from build123d import *

# Parameters (mm, degrees)
F0_W     = 37.5
F0_H     = 30
F1_DEPTH = 60


with BuildPart() as f1:
    # F0 (on Front) → F1 (new body)
    with BuildSketch(Plane.XZ):
        with Locations((-18.75, -15)):
            Rectangle(F0_W, F0_H)
        with Locations((-18.75, 15)):
            Rectangle(F0_W, F0_H)
        with Locations((18.75, 15)):
            Rectangle(F0_W, F0_H)
        with Locations((18.75, -15)):
            Rectangle(F0_W, F0_H)
        Polygon((-75, 0), (-37.5, 0), (-37.5, 30), (0, 30), (0, 60), (-75, 60), align=None)
        Polygon((75, 0), (37.5, 0), (37.5, -30), (0, -30), (0, -60), (75, -60), align=None)
    extrude(amount=F1_DEPTH)


solid = f1.part
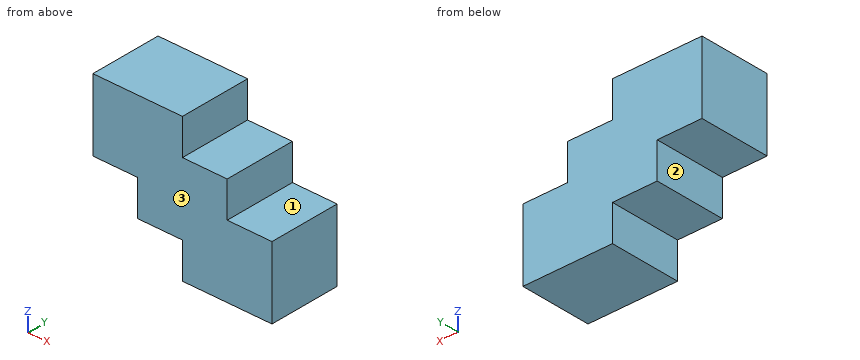
Input: part model. Units: mm. Frame: model coordinates. Face numbers are marked on the shaded views. A direction names the side the tool comes from. Coordinates: 2 decimals unless noted, no trailing zeros. Write each loop counter-clockwise with the first axis right and the second up, starting at its lowest first coordinate (ties: lowest second). Pieces come first, ordered by that corner, then holes. Notation, with made-up numbers: M -19.5,83 L 6.5,83 A24 cw 6.5,103 Z; hole C 28,11.5 d6. An arc over 180 degrees is marked long. Answer as a JSON object with one key per item and string values. Group by question number.
(1) Set-up query: the marked faces 1, 2 and 3. Return all of +Z, -Z, +X, -X, +Y, -Y with unobstructed straight access to the full face (end or side cutting, diameter ignored); none if empty.
(2) Section C-C on x = 24. Output: boundary loops of the cut face in (y, z).
(3) Contact query for flat-ended pins moving along their axis: P1, Ø24, axis at y = -23, z = 41.5, coming from the +X side; P2, Ø8, axis at y = -8, z = -33.5, coming from the -X side; P3, Ø3, axis at y = -20.5, z = 42.5, coming from the +X side. Output: stop coordinate, or through.
(4) Section A-A on y = -19. Output: boundary loops of the cut face in (x, z), plus the area to 4 significant figures.
(5) Ray query, line 1 along Z through (x, y) = (6, -41.5); line 2 along X through (y, z) = (-3, 7.5); line 3 along Z through (x, y) = (-58.5, -7). Return the intervals inside material, ascending. Write a range as [from, to].
(6) Section B-B on z = -49. Output: boundary loops of the cut face in (x, y).
Result set:
{
 "1": {"face 1": "+Z, +X, +Y, -Y", "face 2": "-Z, -X, +Y, -Y", "face 3": "+Z, -Z, +X, -X, -Y"},
 "2": {"outline": "M -60,-60 L 0,-60 L 0,30 L -60,30 Z"},
 "3": {"P1": "stops at x = 37.5", "P2": "stops at x = -37.5", "P3": "stops at x = 0"},
 "4": {"outline": "M -75,0 L -37.5,0 L -37.5,-30 L 0,-30 L 0,-60 L 75,-60 L 75,0 L 37.5,0 L 37.5,30 L 0,30 L 0,60 L -75,60 Z", "area": "11,250 mm2"},
 "5": {"line 1": "z = [-60, 30]", "line 2": "x = [-75, 37.5]", "line 3": "z = [0, 60]"},
 "6": {"outline": "M 0,-60 L 75,-60 L 75,0 L 0,0 Z"}
}
